The listing builds one solid part. Answer for the finished solid, in the listing's coordinates (mm). Give positions to 0.01 mm unless a question says otherwise; leave off trailing zeros. Loops run counter-clockwise (first coordinate to the right, second up) from the corner with the lowest first, then second, coordinate; pieces in that order, holes last. Notation, with made-up numbers: M 45,33.25 L 60,33.25 A21 ccw 60,56.25 Z; hole C 26.5,-22.5 d7. An arc over 180 degrees is marked long. One line per item, written item: value. Start each with the question number.
Q1. A cutting plane is placed at D-D, the plane y = 2.5. Determine the outline of the cut face in (x, z).
Q2. A cutting plane is placed at C-C, the plane x = 23. Determine the outline of the cut face in (y, z), and give its area (3 significant figures).
Q3. A cutting plane is placed at B-B, the plane x = 6. Determine the outline of the cut face in (y, z).
Q4. Consider L1, parallel to X at y = 5, z = 1.75; L2, parallel to X at y = 21, z = 1.3; L3, parallel to X at y = 7.5, z = 2.15. Determine where each line is inside the solid, lowest interval first.
Q5. A cutting plane is placed at A-A, the plane y = 21. Determine the outline of the cut face in (x, z).
Q6. A flat-ended cylindrical pin translates along its axis: pin 1 (8 mm diameter, centred on x = 6, y = 2.5, fed in from -Z). Find the tip coordinate at first contact, or state that the pin passes through.
Autodesk Inventor part; units mm, degrees
ref_plane "XZ Plane" through (0, 0, 0) normal (0, 1, 0) x (-1, 0, 0)
ref_plane "XY Plane" through (0, 0, 0) normal (0, 0, 1) x (1, 0, 0)
sketch "Boceto1" plane through (0, 0, 0) normal (0, 0, 1) x (1, 0, 0)
  line L0 (27.5, -44) -> (-27.5, -44)
  line L1 (-27.5, -44) -> (-27.5, 44)
  line L2 (-27.5, 44) -> (27.5, 44)
  line L3 (27.5, 44) -> (27.5, -44)
  line L4 (27.5, -44) -> (-27.5, 44) construction
  line L5 (-27.5, -44) -> (27.5, 44) construction
  point P0 (0, 0)
  dimension "d0" = 55
  dimension "d1" = 88
extrude "Extrusión1" add sketch "Boceto1" along normal blind 3
sketch "Boceto2" plane through (0, 0, 3) normal (0, 0, 1) x (1, 0, 0)
  line L0 (0, 61.6) -> (0, -61.6) construction
  line L1 (-27.5, -44) -> (27.5, -44) construction
  line L2 (27.5, 44) -> (-27.5, 44) construction
  point P0 (0, 0)
  point P1 (-20, -37)
  point P2 (-10, -37)
  point P3 (20, -37)
  point P4 (10, -37)
  point P5 (-20, 21)
  point P6 (-10, 21)
  point P7 (20, 21)
  point P8 (10, 21)
  dimension "d4" = 10
  dimension "d5" = 0
  dimension "d7" = 10
  dimension "d8" = 7
  dimension "d22" = 23
  dimension "d23" = 10
  dimension "d24" = 0
  dimension "d25" = 10
hole "Agujero1" at (-20, -37, 3) at (-10, -37, 3) at (20, -37, 3) at (10, -37, 3) at (-20, 21, 3) at (-10, 21, 3) at (10, 21, 3) at (20, 21, 3) direction (0, 0, -1) diameter 3 end through all
sketch "Boceto3" plane through (0, 0, 3) normal (0, 0, 1) x (1, 0, 0)
  line L0 (10, -22) -> (-10, -22)
  line L1 (-10, -22) -> (-10, -19)
  line L2 (-10, -19) -> (10, -19)
  line L3 (10, -19) -> (10, -22)
  line L4 (10, -22) -> (-10, -19) construction
  line L5 (-10, -22) -> (10, -19) construction
  line L6 (0, 61.6) -> (0, -61.6) construction
  circle A0 centre (-10, -37) radius 1.5 construction
  line L7 (10, 36) -> (-10, 36)
  line L8 (-10, 36) -> (-10, 39)
  line L9 (-10, 39) -> (10, 39)
  line L10 (10, 39) -> (10, 36)
  line L11 (10, 36) -> (-10, 39) construction
  line L12 (-10, 36) -> (10, 39) construction
  circle A1 centre (-10, 21) radius 1.5 construction
  point P0 (0, 0)
  point P1 (0, -20.5)
  point P2 (0, 37.5)
  point P3 (0, 36)
  dimension "d16" = 3
  dimension "d17" = 20
  dimension "d21" = 15
  dimension "d26" = 3
  dimension "d27" = 20
  dimension "d28" = 15
extrude "Extrusión2" cut sketch "Boceto3" against normal through all
fillet "Empalme1" radius 2 4 edges at (-27.5, -44, 1.5) (27.5, -44, 1.5) (27.5, 44, 1.5) (-27.5, 44, 1.5)
sketch "Boceto5" plane through (0, 0, 3) normal (0, 0, 1) x (1, 0, 0)
  circle A0 centre (-6, 5) radius 1.6 construction
  circle A1 centre (-6, -5) radius 1.6 construction
  circle A2 centre (6, -5) radius 1.6 construction
  circle A3 centre (6, 5) radius 1.6 construction
hole "Agujero2" at (-6, 5, 3) at (-6, -5, 3) at (6, -5, 3) at (6, 5, 3) direction (0, 0, -1) diameter 3 end through all
sketch "Boceto6" plane through (0, 0, 3) normal (0, 0, 1) x (1, 0, 0)
  line L0 (-21, -10) -> (-24, -10)
  line L1 (-24, -10) -> (-24, 10)
  line L2 (-24, 10) -> (-21, 10)
  line L3 (-21, 10) -> (-21, -10)
  line L4 (-38.5, 0) -> (38.5, 0) construction
  line L5 (0, 61.6) -> (0, -61.6) construction
  line L6 (21, -10) -> (24, -10)
  line L7 (24, -10) -> (24, 10)
  line L8 (24, 10) -> (21, 10)
  line L9 (21, 10) -> (21, -10)
  line L10 (-21, 14) -> (-21, -14) construction
  point P0 (0, 0)
  point P1 (-24, 0)
  point P2 (22, -14)
  point P3 (24, 0)
  dimension "d37" = 20
  dimension "d38" = 3
extrude "Extrusión3" cut sketch "Boceto6" against normal through all
properties part number "PlacaFrontalSTD"
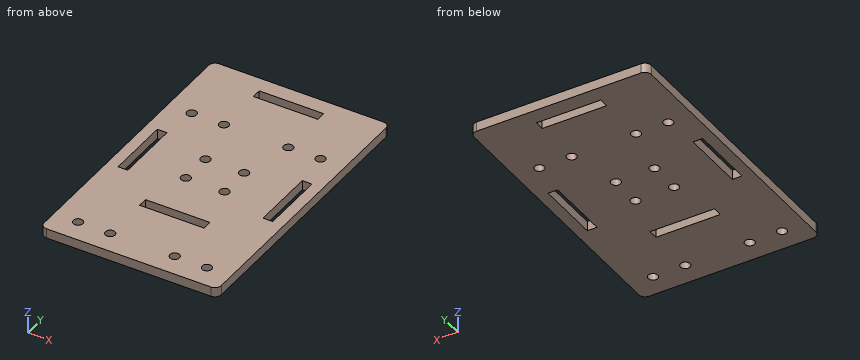
Answer block:
1. outline: M -27.5,0 L -24,0 L -24,3 L -27.5,3 Z; M -21,0 L 21,0 L 21,3 L -21,3 Z; M 24,0 L 27.5,0 L 27.5,3 L 24,3 Z
2. outline: M -44,0 L -10,0 L -10,3 L -44,3 Z; M 10,0 L 44,0 L 44,3 L 10,3 Z
2. area: 204 mm^2
3. outline: M -44,0 L -22,0 L -22,3 L -44,3 Z; M -19,0 L -6.5,0 L -6.5,3 L -19,3 Z; M -3.5,0 L 3.5,0 L 3.5,3 L -3.5,3 Z; M 6.5,0 L 36,0 L 36,3 L 6.5,3 Z; M 39,0 L 44,0 L 44,3 L 39,3 Z
4. L1: -27.5 to -24, -21 to -7.5, -4.5 to 4.5, 7.5 to 21, 24 to 27.5
4. L2: -27.5 to -21.5, -18.5 to -11.5, -8.5 to 8.5, 11.5 to 18.5, 21.5 to 27.5
4. L3: -27.5 to -24, -21 to 21, 24 to 27.5
5. outline: M -27.5,0 L -21.5,0 L -21.5,3 L -27.5,3 Z; M -18.5,0 L -11.5,0 L -11.5,3 L -18.5,3 Z; M -8.5,0 L 8.5,0 L 8.5,3 L -8.5,3 Z; M 11.5,0 L 18.5,0 L 18.5,3 L 11.5,3 Z; M 21.5,0 L 27.5,0 L 27.5,3 L 21.5,3 Z
6. pin 1: z = 0
